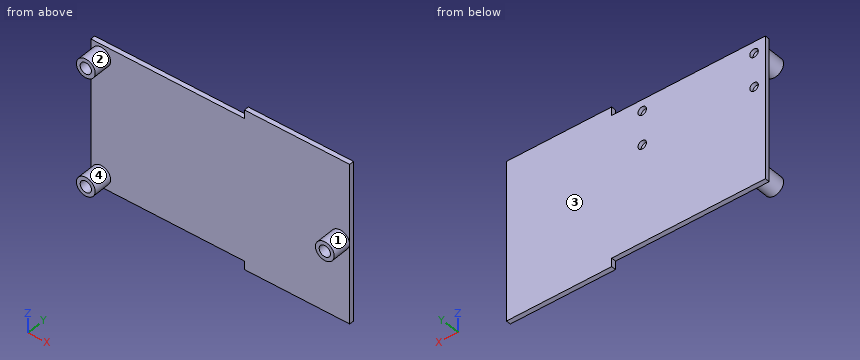
Autodesk Inventor part; units mm, degrees
ref_plane "YZ Plane" through (0, 0, 0) normal (1, 0, 0) x (0, 1, 0)
ref_plane "XZ Plane" through (0, 0, 0) normal (0, 1, 0) x (-1, 0, 0)
ref_plane "XY Plane" through (0, 0, 0) normal (0, 0, 1) x (1, 0, 0)
sketch "Sketch1" plane through (0, 0, 0) normal (0, 1, 0) x (-1, 0, 0)
  line L0 (0, 0) -> (56, 0)
  line L1 (137.742, -4.5) -> (137.742, -80.5)
  line L2 (56, -85) -> (0, -85)
  line L3 (0, -85) -> (0, 0)
  line L4 (0, 0) -> (56, 0)
  line L5 (56, 0) -> (56, -4.5)
  line L6 (56, -85) -> (56, -80.5)
  line L7 (56, -80.5) -> (137.742, -80.5)
  line L8 (56, -4.5) -> (137.742, -4.5)
  line L9 (56, 0) -> (56, -4.5)
  line L10 (56, -80.5) -> (56, -85)
  dimension "d19" = 56
  dimension "d20" = 4.5
  dimension "d21" = 4.5
  dimension "d54" = 76
  dimension "d55" = 81.742
  dimension "d56" = 85
extrude "Extrusion1" add sketch "Sketch1" along normal blind 2.5
sketch "Sketch3" plane through (0, 2.5, 0) normal (0, 1, 0) x (1, 0, 0)
  line L0 (-56, 85) -> (-56, 80.5)
  line L1 (0, 0) -> (0, 85)
  circle A0 centre (-131.742, 10.5) radius 2.2
  line L2 (-137.742, 80.5) -> (-137.742, 4.5)
  line L3 (-137.742, 4.5) -> (-56, 4.5)
  line L4 (-131.742, 10.5) -> (-72.242, 10.5)
  line L5 (-101.992, 10.5) -> (-101.992, 4.5)
  circle A1 centre (-72.242, 10.5) radius 2.2
  line L6 (-72.242, 10.5) -> (-72.242, 28.5)
  circle A2 centre (-72.242, 28.5) radius 2.2
  circle A3 centre (-131.742, 28.5) radius 2.2
  point P0 (-56, 88)
  dimension "d22" = 56
  dimension "d23" = 4.4
  dimension "d24" = 6
  dimension "d25" = 6
  dimension "d26" = 59.5
  dimension "d28" = 18
  dimension "d29" = 4.4
  dimension "d42" = 4.4
  dimension "d43" = 4.4
sketch "Sketch4" plane through (0, 0, 0) normal (0, -1, 0) x (1, 0, 0)
  line L0 (0, 0) -> (0, -85)
  line L1 (0, -42.5) -> (-5.074, -42.5)
  circle A0 centre (-5.074, -42.5) radius 3
  circle A1 centre (-5.074, -42.5) radius 5
  circle A2 centre (-132.242, -74) radius 3
  line L2 (-56, -80.5) -> (-137.742, -80.5)
  line L3 (-137.742, -80.5) -> (-137.742, -4.5)
  circle A3 centre (-132.242, -74) radius 5
  circle A4 centre (-132.242, -11) radius 3
  circle A5 centre (-132.242, -11) radius 5
  line L4 (-137.742, -4.5) -> (-56, -4.5)
  dimension "d33" = 5.074
  dimension "d34" = 6
  dimension "d35" = 10
  dimension "d36" = 6
  dimension "d37" = 6.5
  dimension "d38" = 5.5
  dimension "d39" = 10
  dimension "d57" = 63
  dimension "d58" = 6.5
  dimension "d59" = 5.5
extrude "Extrusion3" add sketch "Sketch4" along normal blind 10
hole "Hole1" at (-72.242, 2.5, -28.5) at (-72.242, 2.5, -10.5) at (-131.742, 2.5, -10.5) at (-131.742, 2.5, -28.5) direction (0, -1, 0) diameter 4.5 depth 2
properties part number "TopChassis"
Work out the finished part from the listing and answer in its coordinate system (mm). Face numbers are marked on the shaded views. Round coordinates to 2 decimals unless told otherwise and drop trailing zeros. Loops run counter-clockwise (first coordinate to the right, second up) from the corner with the lowest first, then second, coordinate; pieces in that order, holes last. Notation, with made-up numbers: M 40.5,61 L 87.5,61 A36 ccw 87.5,100 Z; hole C 25,41 d4. An arc over 180 degrees is marked long. One line per question, with ' | ' between items. Start each with the question number.
(1) For a pull along Z with two mould halves and no side action, classify the marked faces 1, 2, 3 and 4 as released by +Z, released by -Z, zero draft, split by the parting line, or undercut.
(2) A cutting plane is placed at B-B on z = -74. Write down the section's boundary in (x, y).
(3) A cutting plane is placed at C-C on x = -100. Write down the section's boundary in (y, z), plus the area to 3 significant figures.
(4) Find the intervals of material crossed by line 1 (X direction, y = 1.8, z = -10.5); line 2 (Y direction, x = -122, z = -78.5); line 3 (Z direction, x = -66, y = 1), in increasing order.
(5) Flat-ended cylindrical pins translate along their axes: pin 1 Ø1.5 at (y, z) = (-0.5, -30.5) entering from -X; pin 2 Ø1.8 at (x, z) = (-133.5, -73.5) entering from -Y; pin 3 Ø1.3 at (x, z) = (-132.5, -29) entering from +Y; pin 4 Ø5 at (y, z) = (-7, -34) entering from +X. Find the tip coordinate at first contact, or state that the pin passes through.
(6) A cutting plane is placed at A-A on y = -3.5. Write down the section's boundary in (x, z), plus the area to 3 significant figures.
(7) A cutting plane is placed at D-D on z = -28.5. Write down the section's boundary in (x, y), plus the area to 3 significant figures.
Geometry check:
1) face 1: split by the parting line | face 2: undercut | face 3: zero draft | face 4: undercut
2) outline: M -137.74,0 L -137.24,0 L -137.24,-10 L -135.24,-10 L -135.24,0 L -129.24,0 L -129.24,-10 L -127.24,-10 L -127.24,0 L 0,0 L 0,2.5 L -137.74,2.5 Z
3) outline: M 0,-80.5 L 2.5,-80.5 L 2.5,-4.5 L 0,-4.5 Z | area: 190 mm²
4) line 1: x = -137.74 to -133.99, -129.49 to -74.49, -69.99 to 0 | line 2: y = 0 to 2.5 | line 3: z = -80.5 to -4.5
5) pin 1: stops at x = -137.74 | pin 2: stops at y = 0 | pin 3: stops at y = 0.5 | pin 4: passes through
6) outline: C -132.24,-74 d10; C -132.24,-11 d10; C -5.07,-42.5 d10; hole C -132.24,-74 d6; hole C -132.24,-11 d6; hole C -5.07,-42.5 d6 | area: 151 mm²
7) outline: M -137.74,0 L 0,0 L 0,2.5 L -69.99,2.5 L -69.99,0.5 L -74.49,0.5 L -74.49,2.5 L -129.49,2.5 L -129.49,0.5 L -133.99,0.5 L -133.99,2.5 L -137.74,2.5 Z | area: 326 mm²
